For this review, take the finished solid that the model builds, in its own axes (mm). Coordinates: 2 decimals unless noted, no trailing zeros. Order: outer loops, then holes, each group sorted by start corner. A loop starts at its lowest first (then second) coordinate and runs counter-clockwise, first axis right, second up. Notation, with made-up numbers: M 13.5,16 L 23.5,16 A24 cw 23.5,42 Z; hole C 18.25,5.5 d8. An arc over 180 degrees is marked long. Use one line per item in the form item = value. Start each with the question number.
```python
from build123d import *

# Parameters (mm, degrees)
F0_W     = 63.5
F0_H     = 44.45
F1_DEPTH = 12.7
F2_R     = 12.7
F3_R     = 12.7
F4_R     = 12.7
F5_R     = 12.7
F6_R     = 5.08
F7_DEPTH = 25.4


with BuildPart() as f1:
    # F0 (on Front) → F1 (new body)
    with BuildSketch(Plane.XZ):
        with Locations((31.75, 22.225)):
            Rectangle(F0_W, F0_H)
    extrude(amount=F1_DEPTH)

    # F2
    f2_edges = [f1.edges().sort_by_distance(p)[0] for p in [
        (0, -6.35, 44.45),
    ]]
    fillet(f2_edges, radius=F2_R)

    # F3
    f3_edges = [f1.edges().sort_by_distance(p)[0] for p in [
        (63.5, -6.35, 44.45),
    ]]
    fillet(f3_edges, radius=F3_R)

    # F4
    f4_edges = [f1.edges().sort_by_distance(p)[0] for p in [
        (0, -6.35, 0),
    ]]
    fillet(f4_edges, radius=F4_R)

    # F5
    f5_edges = [f1.edges().sort_by_distance(p)[0] for p in [
        (63.5, -6.35, 0),
    ]]
    fillet(f5_edges, radius=F5_R)

    # F6
    f6_edges = [f1.edges().sort_by_distance(p)[0] for p in [
        (59.780256, -12.7, 40.730256),
    ]]
    fillet(f6_edges, radius=F6_R)

    # F7 (add): a face of the model
    f7_faces = [f1.faces().sort_by_distance(p)[0] for p in [
        (31.75, 0, 22.225),
    ]]
    extrude(f7_faces, amount=F7_DEPTH)


solid = f1.part
```
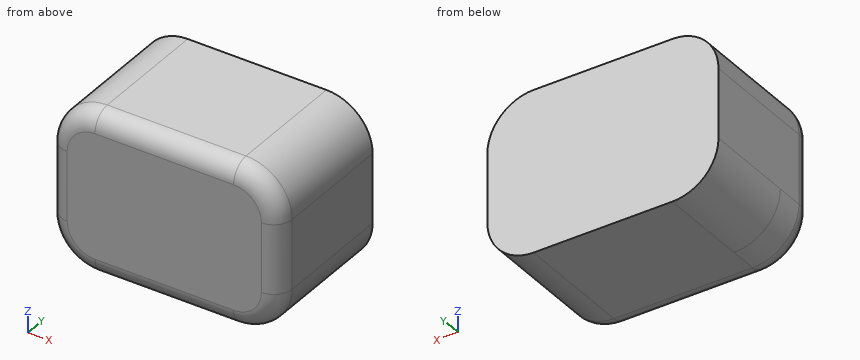
1. To check wall thickness, follow line 1 (Z direction, x = 51, y = -2); line 2 (X direction, y = 8.5, z = 4); line 3 (X direction, y = -9, z = 13). State the ranges of each line that lie inside material, in increasing order.
2. Consider section A-A, the plane y = -1. Write out the cut boundary in (x, z).
3. For pin 1 Ø8 at (x, y) = (57, 4) entering from +Z, flat-tipped, find the tip position at first contact; note if it passes through.
Answers follow:
q1.line_1 = 0 to 44.45
q1.line_2 = 3.45 to 60.05
q1.line_3 = 0.19 to 63.31
q2.outline = M 0,12.7 A12.7 ccw 12.7,0 L 50.8,0 A12.7 ccw 63.5,12.7 L 63.5,31.75 A12.7 ccw 50.8,44.45 L 12.7,44.45 A12.7 ccw 0,31.75 Z
q3.pin_1 = 44.26
